Verification items for this drawing (mm, ordinates from the low corner). A direction names the side the tool comes from. Coordinates: 2 decimals unless noted, no trailing zeros. Order: outer loops, then holes, each group sorted by start corner. A loop starts at its lowest first (then second) coordinate and runs counter-clockwise, first axis right, second up. Notation, with made-up numbers: (86, 42) - (145, 42) arc R14 ccw to (145, 48) - close; hole circle Ø3 at (-17, 35.25). An arc over 180 degrees is marked (long way). Use CSV: the item, a comma, the result in double quotes. Start each with the question number.
1) Tool access check on the marked faces 5 and 6. Record the directions out of +Z, -Z, +X, -X, +Y, -Y that give a thin tool (end or side, any length) a straight path to the whole face; none if there is none.
2) Draft check along Z on the marked faces 1, 2, 3 and 4. Enter one of: released by +Z, released by -Z, zero draft, split by the parting line, or undercut.
3) Sectioned sample at B-B, the plane z = 10.5. Record the cut outline in (x, y), and give its area (3 significant figures).
4) Depth check by flat-ended pin: P1, Ø1.5, axis at x = 28, y = 28.5, coming from the -Z side; P2, Ø12, axis at x = 43, y = 32.5, coming from the +Z side; P3, Ø4, axis at x = 22.5, y = 42.5, coming from the -Z side. Enter the tip coordinate at first touch or a pass-through.
5) Sectioned sample at D-D, the plane z = 38.1. Record the cut outline in (x, y) (1 decimal), and give its area (3 significant figures).
6) Sectioned sample at A-A, the plane x = 25.4. Record the cut outline in (y, z) (1 decimal).
7) Thickness scan on probe 1 along Z at (x, y) = (25, 49) (1 decimal); probe 2 along Y at (x, z) = (9, 59.5); probe 3 along Y at (x, z) = (13, 32). Record the ranges inside material, lowest first. Write a range as [from, to].
8) Sectioned sample at C-C, the plane y = 49.5. Record the cut outline in (x, z) (1 decimal).
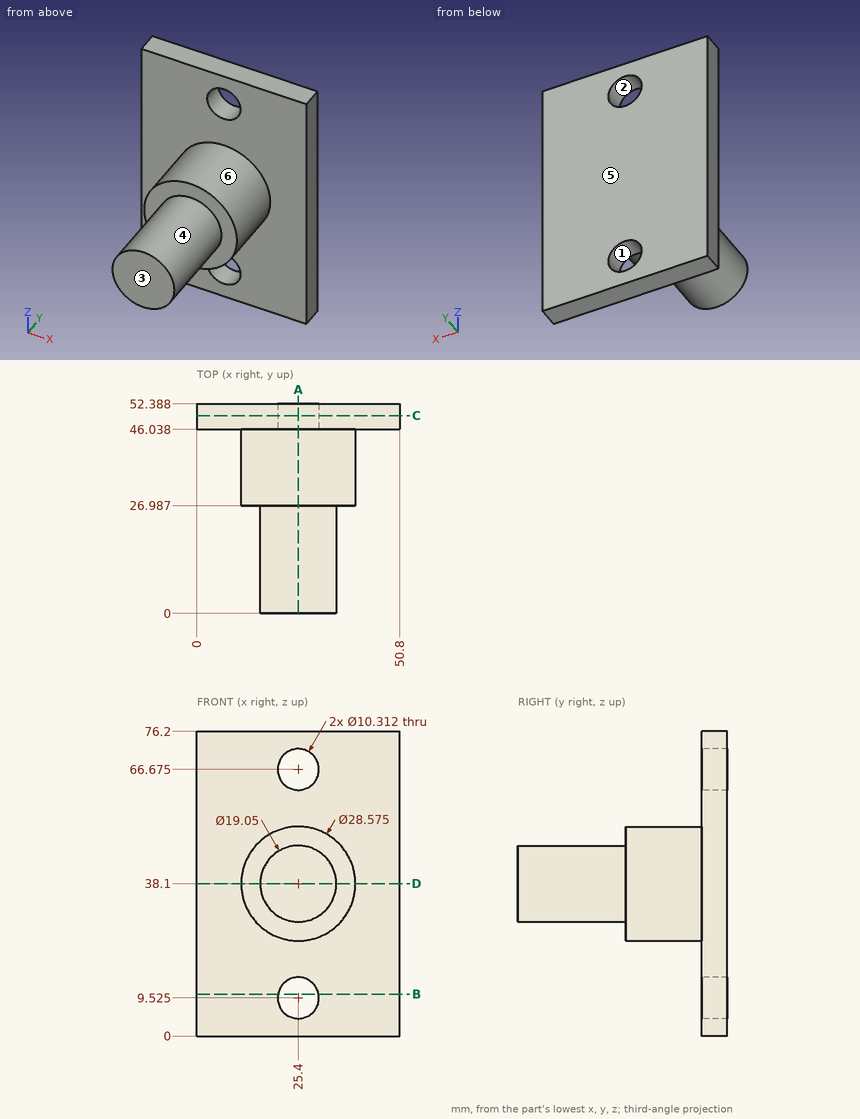
Evaluation:
1,face 5,"+Z, -Z, +X, -X, +Y"
1,face 6,"-Y"
2,face 1,"undercut"
2,face 2,"undercut"
2,face 3,"zero draft"
2,face 4,"split by the parting line"
3,outline,"(0, 46.04) - (20.34, 46.04) - (20.34, 52.39) - (0, 52.39) - close; (30.46, 46.04) - (50.8, 46.04) - (50.8, 52.39) - (30.46, 52.39) - close"
3,area,"258 mm²"
4,P1,"z = 23.93"
4,P2,"z = 46.44"
4,P3,"z = 23.84"
5,outline,"(0, 46) - (11.1, 46) - (11.1, 27) - (15.9, 27) - (15.9, 0) - (34.9, 0) - (34.9, 27) - (39.7, 27) - (39.7, 46) - (50.8, 46) - (50.8, 52.4) - (0, 52.4) - close"
5,area,"1,380 mm²"
6,outline,"(0, 28.6) - (27, 28.6) - (27, 23.8) - (46, 23.8) - (46, 14.7) - (52.4, 14.7) - (52.4, 61.5) - (46, 61.5) - (46, 52.4) - (27, 52.4) - (27, 47.6) - (0, 47.6) - close; (46, 0) - (52.4, 0) - (52.4, 4.4) - (46, 4.4) - close; (46, 71.8) - (52.4, 71.8) - (52.4, 76.2) - (46, 76.2) - close"
7,probe 1,"[0, 4.4], [14.7, 61.5], [71.8, 76.2]"
7,probe 2,"[46.04, 52.39]"
7,probe 3,"[26.99, 52.39]"
8,outline,"(0, 0) - (50.8, 0) - (50.8, 76.2) - (0, 76.2) - close; hole circle Ø10.3 at (25.4, 9.5); hole circle Ø10.3 at (25.4, 66.7)"
